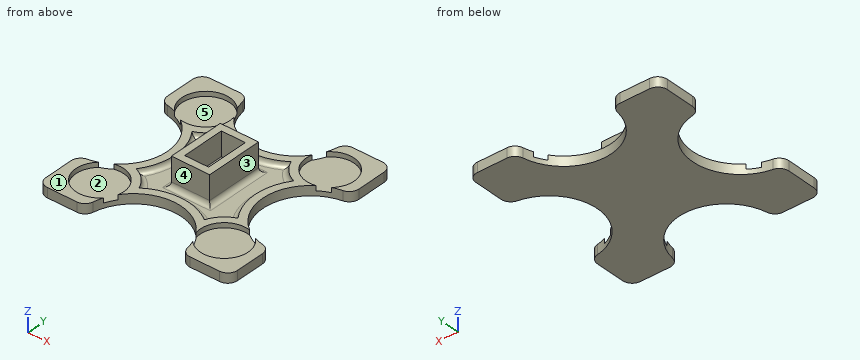
```python
from build123d import *

# Parameters (mm, degrees)
F0_W      = 101.6
F0_H      = 101.6
F1_DEPTH  = 5.08
F2_R      = 12.7
F3_DEPTH  = 2.54
F4_W      = 20.32
F4_H      = 30.48
F4_W_2    = 12.7
F4_H_2    = 22.86
F5_DEPTH  = 12.7
F6_R      = 25.4
F7_DEPTH  = 25.4
F8_R      = 5.08
F9_W      = 20.32
F9_H      = 30.48
F10_DEPTH = 2.54
F11_R     = 2.53999


# Not quite as in the source:
# - a fillet or chamfer is up to 0.001 mm smaller than in the source, because OpenCascade refuses the exact size


with BuildPart() as f1:
    # F0 (on Top) → F1 (new body)
    with BuildSketch(Plane.XY):
        Rectangle(F0_W, F0_H)
    extrude(amount=F1_DEPTH)

    # F2 (on face) → F3 (cut)
    with BuildSketch(Plane.XY.offset(5.08)):
        with Locations((-33.02, 33.02)):
            Circle(F2_R)
        with Locations((33.02, 33.02)):
            Circle(F2_R)
        with Locations((33.02, -33.02)):
            Circle(F2_R)
        with Locations((-33.02, -33.02)):
            Circle(F2_R)
    extrude(amount=-F3_DEPTH, mode=Mode.SUBTRACT)

    # F4 (on face) → F5 (join)
    with BuildSketch(Plane.XY.offset(5.08)):
        Rectangle(F4_W, F4_H)
        Rectangle(F4_W_2, F4_H_2, mode=Mode.SUBTRACT)
    extrude(amount=F5_DEPTH)

    # F6 (on face) → F7 (cut)
    with BuildSketch(Plane.XY.offset(5.08)):
        with Locations((-50.8, 0)):
            Circle(F6_R)
        with Locations((50.8, 0)):
            Circle(F6_R)
        with Locations((0, 50.8)):
            Circle(F6_R)
        with Locations((0, -50.8)):
            Circle(F6_R)
    extrude(amount=-F7_DEPTH, mode=Mode.SUBTRACT)

    # F8
    f8_edges = [f1.edges().sort_by_distance(p)[0] for p in [
        (-50.8, -25.4, 2.54),
        (-50.8, 25.4, 2.54),
        (-50.8, -50.8, 2.54),
        (25.4, -50.8, 2.54),
        (-25.4, -50.8, 2.54),
        (50.8, -50.8, 2.54),
        (50.8, -25.4, 2.54),
        (50.8, 25.4, 2.54),
        (50.8, 50.8, 2.54),
        (-25.4, 50.8, 2.54),
        (25.4, 50.8, 2.54),
        (-50.8, 50.8, 2.54),
    ]]
    fillet(f8_edges, radius=F8_R)

    # F9 (on face) → F10 (cut)
    with BuildSketch(Plane.XY.offset(5.08)):
        with BuildLine():
            ThreePointArc((27.0028755866, -17.3730866956), (21.3360004127, 0), (27.0028755866, 17.3730866956))
            ThreePointArc((27.0028755866, 17.3730866956), (21.166062212, 21.166062212), (17.3730866956, 27.0028755866))
            ThreePointArc((17.3730866956, 27.0028755866), (0, 21.3360004127), (-17.3730866956, 27.0028755866))
            ThreePointArc((-17.3730866956, 27.0028755866), (-21.166062212, 21.166062212), (-27.0028755866, 17.3730866956))
            ThreePointArc((-27.0028755866, 17.3730866956), (-21.3360004127, 0), (-27.0028755866, -17.3730866956))
            ThreePointArc((-27.0028755866, -17.3730866956), (-21.166062212, -21.166062212), (-17.3730866956, -27.0028755866))
            ThreePointArc((-17.3730866956, -27.0028755866), (0, -21.3360004127), (17.3730866956, -27.0028755866))
            ThreePointArc((17.3730866956, -27.0028755866), (21.166062212, -21.166062212), (27.0028755866, -17.3730866956))
        make_face()
        Rectangle(F9_W, F9_H, mode=Mode.SUBTRACT)
    extrude(amount=-F10_DEPTH, mode=Mode.SUBTRACT)

    # F11 (radius 2.54 in the source; OpenCascade refuses exactly that, so slightly less here)
    f11_edges = [f1.edges().sort_by_distance(p)[0] for p in [
        (21.336, 0, 2.54),
        (21.166062, 21.166062, 2.54),
        (0, 21.336, 2.54),
        (-21.166062, 21.166062, 2.54),
        (-21.336, 0, 2.54),
        (-21.166062, -21.166062, 2.54),
        (0, -21.336, 2.54),
        (21.166062, -21.166062, 2.54),
        (-10.16, 0, 2.54),
        (0, 15.24, 2.54),
        (10.16, 0, 2.54),
        (0, -15.24, 2.54),
    ]]
    fillet(f11_edges, radius=F11_R)


solid = f1.part
```
For this review, take the finished solid that the model builds, in its own axes (mm). Face numbers are marked on the shaded views. A direction names the side the tool comes from. Round coordinates to 2 decimals unless told otherwise and drop trailing zeros. Write each loop counter-clockwise with the first axis right and the second up, starting at its lowest first coordinate (ties: lowest second). Pieces come first, ordered by that corner, then holes. Notation, with made-up numbers: (79.5, 60) - (131.5, 60) arc R17 ccw to (131.5, 77) - close; hole circle Ø10 at (20.5, -30). An arc over 180 degrees is marked (long way). Answer as a JSON object with one key per item and string values.
1. We need section B-B on y = 44. Give the boundary of the cut face in (x, z).
Response values:
{"outline": "(-50.8, 0) - (-24.47, 0) - (-24.47, 5.08) - (-26.64, 5.08) - (-26.64, 2.54) - (-39.4, 2.54) - (-39.4, 5.08) - (-50.8, 5.08) - close; (24.47, 0) - (50.8, 0) - (50.8, 5.08) - (39.4, 5.08) - (39.4, 2.54) - (26.64, 2.54) - (26.64, 5.08) - (24.47, 5.08) - close"}
2. Tool access review of the marked faces 1 and 2: name each direction out of +Z, -Z, +X, -X, +Y, -Y from which nothing blocks a thin tool from reaching the whole face with its end or side.
Response values:
{"face 1": "+Z, +X, -X, +Y, -Y", "face 2": "+Z"}
3. Draft analysis for pull direction Y (two halves, no side actions). For the marked faces 3, 4 and 5, state which applies: +Y half, -Y half, draft (parallel to the pull), parting line (faces both ways), or undercut.
Response values:
{"face 3": "draft", "face 4": "-Y half", "face 5": "undercut"}
4. We need section A-A on z = 8.75. Give the boundary of the cut face in (x, y).
Response values:
{"outline": "(-10.16, -15.24) - (10.16, -15.24) - (10.16, 15.24) - (-10.16, 15.24) - close; hole (-6.35, -11.43) - (6.35, -11.43) - (6.35, 11.43) - (-6.35, 11.43) - close"}
5. To check wall thickness, follow line 1 along X through (y, z) = (12.5, 3.75); line 2 along Z through (x, y) = (38.5, -31); line 3 along X through (y, z) = (1, 2). State the ranges of each line that lie inside material, in increasing order.
Response values:
{"line 1": "x = -28.69 to -23.7, -10.54 to 10.54, 23.7 to 28.69", "line 2": "z = 0 to 2.54", "line 3": "x = -25.42 to 25.42"}
6. We need section C-C on x = 33.02. Give the boundary of the cut face in (y, z), then the cut area to 3 significant figures.
Response values:
{"outline": "(-50.8, 0) - (-18.14, 0) - (-18.14, 5.08) - (-20.32, 5.08) - (-20.32, 2.54) - (-45.72, 2.54) - (-45.72, 5.08) - (-50.8, 5.08) - close; (18.14, 0) - (50.8, 0) - (50.8, 5.08) - (45.72, 5.08) - (45.72, 2.54) - (20.32, 2.54) - (20.32, 5.08) - (18.14, 5.08) - close", "area": "203 mm2"}
7. For pin 1 Ø8 at (x, z) = (-12, 11) entering from +Y; pin 2 Ø1.5 at (x, y) = (-27, -17.5) entering from +Z; pin 3 Ø1.5 at (y, z) = (-26, 5.5) entering from +X, all flat-tipped, find the tip position at first contact; note any pin that passes through.
Response values:
{"pin 1": "stops at y = 15.24", "pin 2": "stops at z = 5.08", "pin 3": "stops at x = 49.47"}
